Geometry check sheet. Reference: the model listing, model coordinates, mm. Round coordinates to 2 decimals unless told otherwise and drop trailing zeros. Write each loop counter-clockwise with the first axis right and the second up, starting at its lowest first coordinate (ties: lowest second). Pieces come first, ordered by that corner, then holes. Notation, with made-up numbers: (59, 9.5) - (112, 9.5) arc R29 ccw to (112, 41.5) - close; hole circle Ø2 at (-37, 45.25). An arc over 180 degrees is marked (long way). Return JSON: item names as keys, results as strings. Group by question number.
from build123d import *

# Parameters (mm, degrees)
F0_R     = 12.75
F0_R_2   = 10.25
F1_DEPTH = 3


with BuildPart() as f1:
    # F0 (on Top) → F1 (new body)
    with BuildSketch(Plane.XY):
        Circle(F0_R)
        Circle(F0_R_2, mode=Mode.SUBTRACT)
    extrude(amount=F1_DEPTH)

    # F2 (on Front) → F3 (revolve)
    with BuildSketch(Plane.XZ):
        Polygon((-10.2241979912, 0), (-11.5249808878, 0), (-25.64777527, -22.1678614616), (-24.3469923735, -22.1678614616), align=None)
    revolve(axis=Axis((-18.5863780789, 0, -11.0839307308), (0.5373079732, 0, 0.8433861168)))


solid = f1.part
1. Section check A-A (x = 0). Enter the section's corners in (y, z), and give its area (3 significant figures).
2. Depth check by flat-ended pin: pin 1 Ø12 at (x, y) = (-14, -1.5) entering from -Z; pin 2 Ø1.5 at (y, z) = (1.5, -2) entering from -X. Enter the tip coordinate at first touch or a pass-through.
3. Mould release check, pull along X, two halves, no side actions. Record for faces 1 (the face through (-2.764, -12.447, 1.479)), 2 (the face through (-2.222, -10.006, 1.479)), 3 (the face through (-25.71, -0.12, -21.98)): pulls with the +X half, pulls with the -X half, needs draft (parallel to the pull), parting line crosses it, or undercut.
4. Material ranges on line 1 along Y through (x, z) = (0, 1.8); line 2 along X through (y, z) = (-6.25, 1), recorded low to high.
5. Section check B-B (y = -6.5). Enter the section's corners in (x, z).
6. Section check C-C (y = 11.25). Enter the section's corners in (x, z).
Result sheet:
{
 "1": {"outline": "(-12.75, 0) - (-10.25, 0) - (-10.25, 3) - (-12.75, 3) - close; (10.25, 0) - (12.75, 0) - (12.75, 3) - (10.25, 3) - close", "area": "15.0 mm²"},
 "2": {"pin 1": "stops at z = -15.09", "pin 2": "stops at x = -13.86"},
 "3": {"face 1": "parting line crosses it", "face 2": "undercut", "face 3": "pulls with the -X half"},
 "4": {"line 1": "y = -12.75 to -10.25, 10.25 to 12.75", "line 2": "x = -11.11 to -8.12, 8.12 to 11.11"},
 "5": {"outline": "(-10.97, 0) - (-7.93, 0) - (-7.93, 3) - (-10.97, 3) - close; (7.93, 0) - (10.97, 0) - (10.97, 3) - (7.93, 3) - close"},
 "6": {"outline": "(-6, 0) - (6, 0) - (6, 3) - (-6, 3) - close"}
}
